from build123d import *

# Parameters (mm, degrees)
ESQUISSE1_R                  = 10
ESQUISSE1_R_2                = 4
BOSS_EXTRU_1_DEPTH           = 1
ESQUISSE2_R                  = 1.9
ENL_V_MAT_EXTRU_1_DEPTH      = 1
ENL_V_MAT_EXTRU_1_DEPTH_BACK = 2


with BuildPart() as part:
    # Esquisse1 → Boss.-Extru.1 (new body)
    with BuildSketch(Plane.XY):
        Circle(ESQUISSE1_R)
        Circle(ESQUISSE1_R_2, mode=Mode.SUBTRACT)
    extrude(amount=BOSS_EXTRU_1_DEPTH)

    # Esquisse2 → Enlèv. mat.-Extru.1 (cut, two sides)
    with BuildSketch(Plane.XY.offset(1)) as enl_v_mat_extru_1_sk:
        with Locations((7, 0)):
            Circle(ESQUISSE2_R)
        with Locations((0, -7)):
            Circle(ESQUISSE2_R)
        with Locations((-7, 0)):
            Circle(ESQUISSE2_R)
        with Locations((0, 7)):
            Circle(ESQUISSE2_R)
    extrude(amount=ENL_V_MAT_EXTRU_1_DEPTH, mode=Mode.SUBTRACT)
    extrude(enl_v_mat_extru_1_sk.sketch, amount=-ENL_V_MAT_EXTRU_1_DEPTH_BACK, mode=Mode.SUBTRACT)


solid = part.part
The model under review builds one solid part; all positions refer to its coordinate system, in mm. Give positions to 0.01 mm unless a question says otherwise; leave off trailing zeros. Order: outer loops, then holes, each group sorted by start corner. A loop starts at its lowest first (then second) coordinate and runs counter-clockwise, first axis right, second up. Notation, with made-up numbers: M -23,39 L 7,39 A19 ccw 7,62 Z; hole C -37.5,-3 d8. An arc over 180 degrees is marked long. Answer in a Markdown table with one row per item. Add a question column.
1. For pin 1 Ø2.5 at (x, y) = (0, -7) entering from -Z, flat-tipped, find the tip position at first contact; note if it passes through.
2. Mouldability with a two-part tool opening along X and no side actions: class faces 1 (the flat face through (4.3, 0.1, 1)), 2 (the cylindrical face through (5.1, 0.08, 0.51)), 3 (the cylindrical face through (-2.17, -9.76, 0.49)) as released by +X, released by -X, zero draft, split by the parting line, or undercut.
3. Add section A-A on y = 0. State the section outline as (x, z) points, plus the area to 3 significant figures.
4. To check wall thickness, follow line 1 along Y through (x, z) = (0, 0.25); line 2 along X through (y, z) = (-0.5, 0.8); line 3 along X through (y, z) = (0.25, 0.65). State the ranges of each line that lie inside material, in increasing order.
5. Add section C-C on z = 0.5. State the section outline as (x, y) points, plus the area to 3 significant figures.
6. Add section D-D on y = -3.25. State the section outline as (x, z) points.
The answers:
| question | item | result |
|---|---|---|
| 1 | pin 1 | through |
| 2 | face 1 | zero draft |
| 2 | face 2 | undercut |
| 2 | face 3 | split by the parting line |
| 3 | outline | M -10,0 L -8.9,0 L -8.9,1 L -10,1 Z; M -5.1,0 L -4,0 L -4,1 L -5.1,1 Z; M 4,0 L 5.1,0 L 5.1,1 L 4,1 Z; M 8.9,0 L 10,0 L 10,1 L 8.9,1 Z |
| 3 | area | 4.40 mm2 |
| 4 | line 1 | -10 to -8.9, -5.1 to -4, 4 to 5.1, 8.9 to 10 |
| 4 | line 2 | -9.99 to -8.83, -5.17 to -3.97, 3.97 to 5.17, 8.83 to 9.99 |
| 4 | line 3 | -10 to -8.88, -5.12 to -3.99, 3.99 to 5.12, 8.88 to 10 |
| 5 | outline | C 0,0 d20; hole C -7,0 d3.8; hole C 0,0 d8; hole C 0,-7 d3.8; hole C 0,7 d3.8; hole C 7,0 d3.8 |
| 5 | area | 219 mm2 |
| 6 | outline | M -9.46,0 L -2.33,0 L -2.33,1 L -9.46,1 Z; M 2.33,0 L 9.46,0 L 9.46,1 L 2.33,1 Z |
